Work out the finished part from the listing and answer in its coordinate system (mm). A direction names the side the tool comes from. Give positions to 0.01 mm unless a question says otherwise; leave off trailing zeros. Loops run counter-clockwise (first coordinate to the right, second up) from the corner with the lowest first, then second, coordinate; pieces in that order, holes last. Notation, with made-up numbers: M 77.25,32.25 L 82.25,32.25 A22 ccw 82.25,52.25 Z; hole C 19.5,30.5 d3. An arc over 180 degrees is marked long. Use a Markdown table: item, result.
```python
from build123d import *

# Parameters (mm, degrees)
SKETCH1_W           = 63.5
SKETCH1_H           = 63.5
BOSS_EXTRUDE1_DEPTH = 2.54
SKETCH2_W           = 6.35
SKETCH2_H           = 6.35
BOSS_EXTRUDE2_DEPTH = 6.35
FILLET1_R           = 3.175


with BuildPart() as part:
    # Sketch1 → Boss-Extrude1 (new body)
    with BuildSketch(Plane(origin=(0, 0, 0), x_dir=(1, 0, 0), z_dir=(0, 1, 0))):
        with Locations((31.75, 31.75)):
            Rectangle(SKETCH1_W, SKETCH1_H)
    extrude(amount=BOSS_EXTRUDE1_DEPTH)

    # Sketch2 → Boss-Extrude2 (add)
    with BuildSketch(Plane(origin=(0, 2.54, 0), x_dir=(1, 0, 0), z_dir=(0, 1, 0))):
        with Locations((3.175, 3.175)):
            Rectangle(SKETCH2_W, SKETCH2_H)
        with Locations((60.325, 3.175)):
            Rectangle(SKETCH2_W, SKETCH2_H)
        with Locations((3.175, 60.325)):
            Rectangle(SKETCH2_W, SKETCH2_H)
        with Locations((60.325, 60.325)):
            Rectangle(SKETCH2_W, SKETCH2_H)
    extrude(amount=BOSS_EXTRUDE2_DEPTH)

    # Fillet1
    fillet1_edges = [part.edges().sort_by_distance(p)[0] for p in [
        (3.175, 8.89, -6.35),
        (3.175, 8.89, 0),
        (60.325, 8.89, 0),
        (60.325, 8.89, -6.35),
        (60.325, 8.89, -63.5),
        (60.325, 8.89, -57.15),
        (3.175, 8.89, -63.5),
        (3.175, 8.89, -57.15),
    ]]
    fillet(fillet1_edges, radius=FILLET1_R - 0.0001)  # a hair under: the kernel refuses the full size


solid = part.part
```
(1) The mould has two halves that part along X. Classify faces 4 (the flat face through (0, 2, -31)), 5 (the flat face through (31, 2, -63.5)), 6 (the flat face through (6.35, 6, -60)): released by +X, released by -X, zero draft, split by the parting line, or undercut.
Entries:
| item | result |
|---|---|
| face 4 | released by -X |
| face 5 | zero draft |
| face 6 | undercut |
(2) Which of the six approach directions +Z, -Z, +X, -X, +Y, -Y give full straight-line access (tool end or side, diameter ignored) to faces 1 (the cylindrical face through (3.22, 7.98, -58.1)), 2 (the cylindrical face through (60.37, 7.98, -62.55)), 3 (the flat face through (6.35, 6, -3))?
Entries:
| item | result |
|---|---|
| face 1 | +X, -X, +Y |
| face 2 | -Z, +X, -X, +Y |
| face 3 | +Z, -Z, +Y |
(3) Consider probe 1 along Z at (x, y) = (3.5, 3.25); probe 2 along X at (y, z) = (5.5, -58); probe 3 along Y at (x, z) = (35, -20). Determine where each line is inside the solid, lowest interval first. Write a range as [from, to].
Entries:
| item | result |
|---|---|
| probe 1 | z = [-63.5, -57.15], [-6.35, 0] |
| probe 2 | x = [0, 6.35], [57.15, 63.5] |
| probe 3 | y = [0, 2.54] |
(4) A cutting plane is placed at D-D (z = -9.5). Write down the section's boundary in (x, y).
Entries:
| item | result |
|---|---|
| outline | M 0,0 L 63.5,0 L 63.5,2.54 L 0,2.54 Z |
(5) A cutting plane is placed at A-A (y = 3.75). Write down the section's boundary in (x, z).
Entries:
| item | result |
|---|---|
| outline | M 0,-63.5 L 6.35,-63.5 L 6.35,-57.15 L 0,-57.15 Z; M 0,-6.35 L 6.35,-6.35 L 6.35,0 L 0,0 Z; M 57.15,-63.5 L 63.5,-63.5 L 63.5,-57.15 L 57.15,-57.15 Z; M 57.15,-6.35 L 63.5,-6.35 L 63.5,0 L 57.15,0 Z |
(6) A cutting plane is placed at C-C (y = 7). Write down the section's boundary in (x, z).
Entries:
| item | result |
|---|---|
| outline | M 0,-63.23 L 6.35,-63.23 L 6.35,-57.42 L 0,-57.42 Z; M 0,-6.08 L 6.35,-6.08 L 6.35,-0.27 L 0,-0.27 Z; M 57.15,-63.23 L 63.5,-63.23 L 63.5,-57.42 L 57.15,-57.42 Z; M 57.15,-6.08 L 63.5,-6.08 L 63.5,-0.27 L 57.15,-0.27 Z |
